Check sheet for the drawn part. Datum: minimum x, y, z corner. Units: mm. A direction names the side the tool comes from. Give positions to 0.01 mm unless a question says otherwise; leave off trailing zeros. Write each loop counter-clockwise with the first axis right and the second up, starting at its lowest first coordinate (ties: lowest second). Pieces come first, ordered by that corner, then holes. Notation, with made-up numbers: (-36.75, -31) - (-25.75, -31) arc R35 cw to (-25.75, 2) - close; hole circle Ø1 at (38, 44). An arc over 180 degrees is marked (long way). Answer as a JSON object with one key per item and string values. Group by question number.
Item 1: Sectioned sample at C-C, the plane y = 10. Record the boundary of the cut face in (x, z), and give its area (3 significant figures).
Item 2: Scan lines: line 1 along Y through (x, z) = (60, 62); line 2 along X through (y, z) = (11.5, 70.5); line 3 along X through (y, z) = (7.25, 4). Record each from-to range of solid material in increasing order. Write a range as [from, to].
Item 3: Sectioned sample at A-A, the plane x = 60. Record the boundary of the cut face in (y, z).
Item 4: Go/stop test with flat-tipped pins: pin 1 (10 mm diameter, centred on x = 15, z = 66, fed in from -Y); pin 2 (6.5 mm diameter, centred on x = 60, y = 10, fed in from -Z); pin 3 (10 mm diameter, centred on x = 63.5, y = 8.5, fed in from -Z); pin 4 (10 mm diameter, centred on y = 8.5, z = 11, fed in from +X). Record where each tip stops, or that it passes through.
Item 5: Sectioned sample at B-B, the plane z = 20. Record the boundary of the cut face in (x, y).
Item 6: Tool access check on the marked faces 1 and 2. Record the directions out of +Z, -Z, +X, -X, +Y, -Y that give a thin tool (end or side, any length) a straight path to the whole face; none if there is none.
Item 7: Sectioned sample at D-D, the plane x = 39. Record the boundary of the cut face in (y, z).
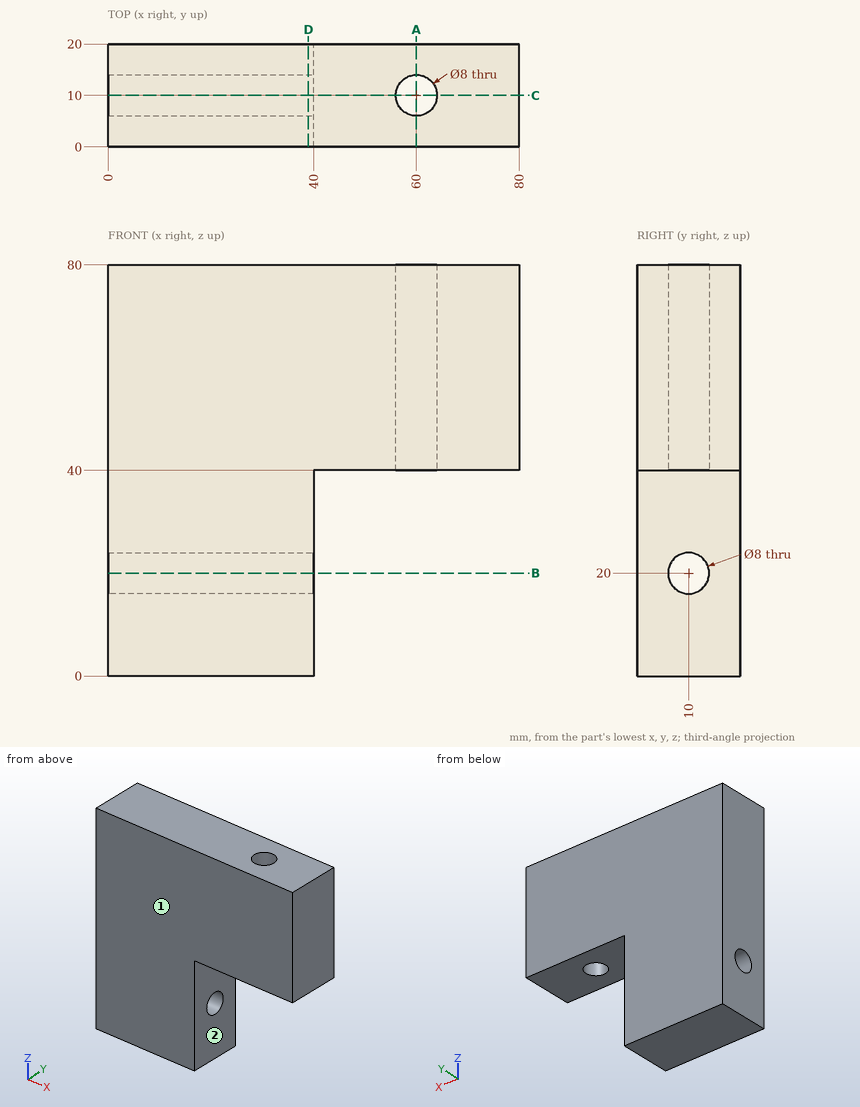
Geometry check:
{
 "1": {"outline": "(0, 0) - (40, 0) - (40, 16) - (0, 16) - close; (0, 24) - (40, 24) - (40, 40) - (56, 40) - (56, 80) - (0, 80) - close; (64, 40) - (80, 40) - (80, 80) - (64, 80) - close", "area": "4,160 mm^2"},
 "2": {"line 1": "[0, 6], [14, 20]", "line 2": "[0, 56.29], [63.71, 80]", "line 3": "[0, 40]"},
 "3": {"outline": "(0, 40) - (6, 40) - (6, 80) - (0, 80) - close; (14, 40) - (20, 40) - (20, 80) - (14, 80) - close"},
 "4": {"pin 1": "y = 0", "pin 2": "through", "pin 3": "z = 40", "pin 4": "x = 40"},
 "5": {"outline": "(0, 0) - (40, 0) - (40, 6) - (0, 6) - close; (0, 14) - (40, 14) - (40, 20) - (0, 20) - close"},
 "6": {"face 1": "+Z, -Z, +X, -X, -Y", "face 2": "-Z, +X, +Y, -Y"},
 "7": {"outline": "(0, 0) - (20, 0) - (20, 80) - (0, 80) - close; hole circle Ø8 at (10, 20)"}
}
